The listing builds one solid part. Answer for the finished solid, in the listing's coordinates (mm). Give positions to 0.01 mm unless a question says otherwise; leave off trailing zeros. Order: outer loops, then holes, each group sorted by start corner. A loop starts at its lowest first (then second) coordinate and runs counter-clockwise, first axis right, second up. Notation, with made-up numbers: (18, 61.5) - (29, 61.5) arc R29 cw to (29, 84.5) - close; hole circle Ø11 at (-35, 32). An arc over 180 degrees is marked (long way). Answer as a JSON object with one key per item and string values. Group by question number.
Q1. Given pin 1 (1.5 mm diameter, centred on x = 52, y = 1.5, fed in from -Z), flat-ended and moving along its own axis, determine where the tip first touches the part or whether it passes through.
Q2. Consider line 1 (X direction, y = 1.85, z = -17.5); line 2 (Z direction, x = 49.5, y = 0.65); line 3 (X direction, y = 2.45, z = 6). Determine where each line is inside the solid, lowest interval first.
Q3. A cutting plane is placed at B-B, the plane z = 6.35. Give the vertices of the cut face in (x, y).
Q4. A cutting plane is placed at A-A, the plane y = 0.45. Give the vertices of the cut face in (x, z), and give its area (3 significant figures).
Q5. The mould has two halves that part along Z. Classify faces 1 (the face through (-89, 1.5, 6.3)), 2 (the face through (89, 1.5, 6.4)), 3 (the face through (1, 3, 0)), 4 (the face through (-97.594, 1.479, 17.719)): released by +Z, released by -Z, zero draft, split by the parting line, or undercut.
Q6. A cutting plane is placed at C-C, the plane x = 53. Give the vertices of the cut face in (y, z).
from build123d import *

# Parameters (mm, degrees)
SKETCH1_W           = 12.7
SKETCH1_H           = 12.7
BOSS_EXTRUDE1_DEPTH = 3


with BuildPart() as part:
    # Sketch1 → Boss-Extrude1 (new body)
    # profile 1 of 2: a face of its own
    with BuildSketch(Plane(origin=(0, 0, 0), x_dir=(1, 0, 0), z_dir=(0, 1, 0))):
        with BuildLine():
            ThreePointArc((-92, -20), (-97.656854249, -17.656854249), (-100, -12))
            Line((-100, -12), (-100, 20))
            Line((-100, 20), (-87.3, 20))
            Line((-87.3, 20), (-87.3, 7.3))
            Line((-87.3, 7.3), (87.3, 7.3))
            Line((87.3, 7.3), (87.3, 20))
            Line((87.3, 20), (100, 20))
            Line((100, 20), (100, -12))
            ThreePointArc((100, -12), (97.656854249, -17.656854249), (92, -20))
            Line((92, -20), (-92, -20))
        make_face()
        with BuildLine():
            ThreePointArc((85, -10.35), (89, -6.35), (85, -2.35))
            Line((85, -2.35), (-85, -2.35))
            ThreePointArc((-85, -2.35), (-89, -6.35), (-85, -10.35))
            Line((-85, -10.35), (85, -10.35))
        make_face(mode=Mode.SUBTRACT)
    # profile 2 of 2: a face of its own
    with BuildSketch(Plane(origin=(0, 0, 0), x_dir=(1, 0, 0), z_dir=(0, 1, 0))):
        with Locations((0, 13.65)):
            Rectangle(SKETCH1_W, SKETCH1_H)
    extrude(amount=BOSS_EXTRUDE1_DEPTH)


solid = part.part
Reply:
{
 "1": {"pin 1": "stops at z = -7.3"},
 "2": {"line 1": "x = -100 to -87.3, -6.35 to 6.35, 87.3 to 100", "line 2": "z = -7.3 to 2.35, 10.35 to 20", "line 3": "x = -100 to -88.98, 88.98 to 100"},
 "3": {"outline": "(-100, 0) - (-89, 0) - (-89, 3) - (-100, 3) - close; (89, 0) - (100, 0) - (100, 3) - (89, 3) - close"},
 "4": {"outline": "(-100, -20) - (-87.3, -20) - (-87.3, -7.3) - (-6.35, -7.3) - (-6.35, -20) - (6.35, -20) - (6.35, -7.3) - (87.3, -7.3) - (87.3, -20) - (100, -20) - (100, 12) arc R8 ccw to (92, 20) - (-92, 20) arc R8 ccw to (-100, 12) - close; hole (-85, 2.35) - (85, 2.35) arc R4 ccw to (85, 10.35) - (-85, 10.35) arc R4 ccw to start", "area": "4,510 mm^2"},
 "5": {"face 1": "undercut", "face 2": "undercut", "face 3": "zero draft", "face 4": "released by +Z"},
 "6": {"outline": "(0, -7.3) - (3, -7.3) - (3, 2.35) - (0, 2.35) - close; (0, 10.35) - (3, 10.35) - (3, 20) - (0, 20) - close"}
}
